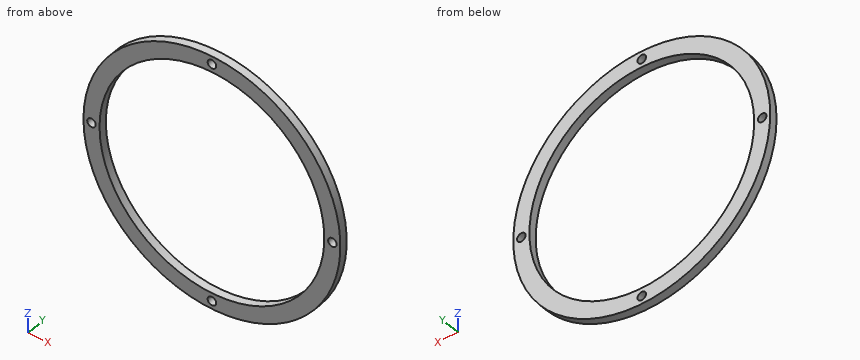
Autodesk Inventor part; units mm, degrees
ref_plane "YZ Plane" through (0, 0, 0) normal (1, 0, 0) x (0, 1, 0)
ref_plane "XZ Plane" through (0, 0, 0) normal (0, 1, 0) x (-1, 0, 0)
ref_plane "XY Plane" through (0, 0, 0) normal (0, 0, 1) x (1, 0, 0)
sketch "Sketch1" plane through (0, 0, 0) normal (0, 1, 0) x (-1, 0, 0)
  circle A0 centre (0, 0) radius 88.9
  circle A1 centre (0, 0) radius 101.6
  circle A2 centre (0, 0) radius 95.25 construction
  circle A3 centre (0, 95.25) radius 3.3782
  circle A4 centre (-95.25, 0) radius 3.3782
  circle A5 centre (0, -95.25) radius 3.3782
  circle A6 centre (95.25, 0) radius 3.3782
  dimension "d2" = 190.5
  dimension "d0" = 177.8
  dimension "d1" = 203.2
  dimension "d3" = 6.7564
  dimension "d6" = 360
extrude "Extrusion1" add sketch "Sketch1" along normal blind 6.35
properties part number "Flywheel Spacer" material "Aluminum 6061"
Design review of the part built by this model. Coordinates are the model's own, in mm. Coordinates: 2 decimals unless noted, no trailing zeros. Loops run counter-clockwise (first coordinate to the right, second up) from the corner with the lowest first, then second, coordinate; pieces in that order, holes last. Notation, with made-up numbers: (4.5, 72) -> (54.5, 72) arc R23 ccw to (54.5, 92) -> close; hole circle Ø11 at (53, -12.75). An arc over 180 degrees is marked (long way). Use a Markdown table: item, result. Add a question column.
Item 1: We need section D-D, the plane x = -38.5. Write out the cut boundary in (y, z), and give its area (3 significant figures).
Item 2: Wall thickness on L1, parallel to Z at x = 0, y = 3.75; L2, parallel to X at y = 5.75, z = 25.5; L3, parallel to Z at x = -14.5, y = 1.75: over which ranges is each line inside the solid? List them lowest first. Write a range as from..to.
Item 3: We need section A-A, the plane x = 0. Write out the cut boundary in (y, z), and give its area (3 significant figures).
Item 4: We need section C-C, the plane y = 3.5. Write out the cut boundary in (x, z).
Item 5: We need section B-B, the plane z = 58.5. Write out the cut boundary in (x, y), and give its area (3 significant figures).
Item 6: Clearance check with flat-ended pins moving along their axes: P1, Ø2, axis at y = 1.5, z = 40, coming from the -X side; P2, Ø11, axis at x = -95.25, z = 0, coming from the +Y side; P3, Ø3, axis at y = 2, z = -9, coming from the +X side; P4, Ø3, axis at y = 1, z = -16, coming from the +X side. State where each tip first meets the part, or that it passes through.
Numbers:
| question | item | result |
|---|---|---|
| 1 | outline | (0, -94.02) -> (6.35, -94.02) -> (6.35, -80.13) -> (0, -80.13) -> close; (0, 80.13) -> (6.35, 80.13) -> (6.35, 94.02) -> (0, 94.02) -> close |
| 1 | area | 176 mm^2 |
| 2 | L1 | z = -101.6..-98.63, -91.87..-88.9, 88.9..91.87, 98.63..101.6 |
| 2 | L2 | x = -98.35..-85.16, 85.16..98.35 |
| 2 | L3 | z = -100.56..-87.71, 87.71..100.56 |
| 3 | outline | (0, -101.6) -> (6.35, -101.6) -> (6.35, -98.63) -> (0, -98.63) -> close; (0, -91.87) -> (6.35, -91.87) -> (6.35, -88.9) -> (0, -88.9) -> close; (0, 88.9) -> (6.35, 88.9) -> (6.35, 91.87) -> (0, 91.87) -> close; (0, 98.63) -> (6.35, 98.63) -> (6.35, 101.6) -> (0, 101.6) -> close |
| 3 | area | 75.5 mm^2 |
| 4 | outline | circle Ø203.2 at (0, 0); hole circle Ø6.76 at (-95.25, 0); hole circle Ø177.8 at (0, 0); hole circle Ø6.76 at (0, -95.25); hole circle Ø6.76 at (0, 95.25); hole circle Ø6.76 at (95.25, 0) |
| 5 | outline | (-83.07, 0) -> (-66.94, 0) -> (-66.94, 6.35) -> (-83.07, 6.35) -> close; (66.94, 0) -> (83.07, 0) -> (83.07, 6.35) -> (66.94, 6.35) -> close |
| 5 | area | 205 mm^2 |
| 6 | P1 | stops at x = -93.82 |
| 6 | P2 | stops at y = 6.35 |
| 6 | P3 | stops at x = 101.32 |
| 6 | P4 | stops at x = 100.56 |
